```python
from build123d import *

# Parameters (mm, degrees)
BOSS_EXTRUDE1_DEPTH                                 = 10
CBORE_FOR_M5_HEX_SOCKET_HEAD_CAP_SCREW1_D           = 5.5
CBORE_FOR_M5_HEX_SOCKET_HEAD_CAP_SCREW1_CBORE_D     = 10
CBORE_FOR_M5_HEX_SOCKET_HEAD_CAP_SCREW1_CBORE_DEPTH = 8


with BuildPart() as part:
    # Sketch1 → Boss-Extrude1 (new, symmetric)
    with BuildSketch(Plane.XY):
        with BuildLine():
            Line((-15, 7.5), (-15, -7.5))
            Line((-15, -7.5), (15, -7.5))
            Line((15, -7.5), (15, 7.5))
            ThreePointArc((15, 7.5), (0, 22.5), (-15, 7.5))
        make_face()
    extrude(amount=BOSS_EXTRUDE1_DEPTH, both=True)

    # CBORE for M5 Hex Socket Head Cap Screw1 (through all)
    with Locations(Plane(origin=(0, 22.5, 0), x_dir=(1, 0, 0), z_dir=(0, 1, 0))):
        with Locations((0, 0)):
            CounterBoreHole(CBORE_FOR_M5_HEX_SOCKET_HEAD_CAP_SCREW1_D / 2, CBORE_FOR_M5_HEX_SOCKET_HEAD_CAP_SCREW1_CBORE_D / 2, CBORE_FOR_M5_HEX_SOCKET_HEAD_CAP_SCREW1_CBORE_DEPTH)


solid = part.part
```
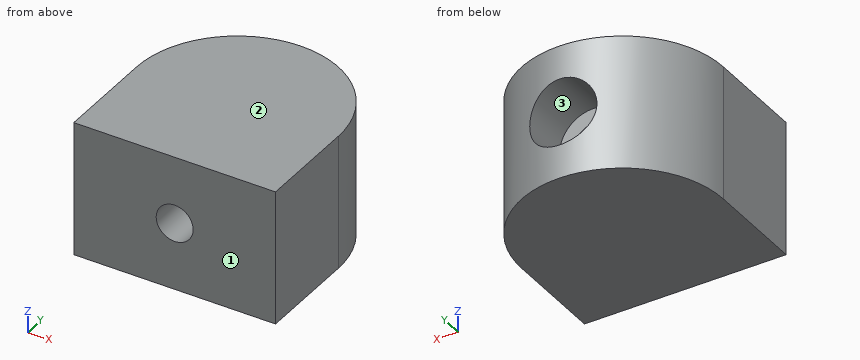
Can you work these out from the model? Positions are in its coordinate system, mm. Face numbers are marked on the shaded views. Coordinates: 2 decimals unless noted, no trailing zeros. Loops run counter-clockwise (first coordinate to the right, second up) from the corner with the lowest first, then second, coordinate; pieces in that order, holes last.
1) I need wall thicknesses on probe 1 along Z at (x, y) = (0, 8.5); probe 2 along Z at (x, y) = (0, 19); probe 3 along X at (y, z) = (16.5, -0.75). Which ranges of each line are inside material? Lowest first, please.
2) Thinking about a two-plate mould opening in Z: for the marked faces 1, 2 and 3, which applies, pulls with the +Z half, pulls with the -Z half, needs draft (parallel to the pull), parting line crosses it, or undercut?
3) For pin 1 (8 mm diameter, centred on x = -2.5, z = 0.5, fed in from +Y), with a flat end and sliding along its axis, tell me the tip position at first contact or that it passes through.
4) Imagine slicing it at B-B on y = -2. List the corners of the cut face in (x, z) for me.
5) Imagine slicing it at C-C on z = -0.5. List the corners of the cut face in (x, y) for me, plus the area to 3 significant figures.
6) Imagine slicing it at D-D on x = -3.5. List the corners of the cut face in (y, z) for me, plus the area to 3 significant figures.
7) Imagine slicing it at A-A on x = 0. List the corners of the cut face in (y, z) for me, plus the area to 3 significant figures.
Completed:
1. probe 1: z = -10 to -2.75, 2.75 to 10
1. probe 2: z = -10 to -5, 5 to 10
1. probe 3: x = -12 to -4.94, 4.94 to 12
2. face 1: needs draft
2. face 2: pulls with the +Z half
2. face 3: undercut
3. pin 1: stops at y = 22.34
4. outline: (-15, -10) - (15, -10) - (15, 10) - (-15, 10) - close; hole circle Ø5.5 at (0, 0)
5. outline: (-15, -7.5) - (-2.7, -7.5) - (-2.7, 14.5) - (-4.97, 14.5) - (-4.97, 21.65) arc R15 ccw to (-15, 7.5) - close; (2.7, -7.5) - (15, -7.5) - (15, 7.5) arc R15 ccw to (4.97, 21.65) - (4.97, 14.5) - (2.7, 14.5) - close
5. area: 608 mm2
6. outline: (-7.5, -10) - (22.09, -10) - (22.09, -3.57) - (14.5, -3.57) - (14.5, 3.57) - (22.09, 3.57) - (22.09, 10) - (-7.5, 10) - close
6. area: 538 mm2
7. outline: (-7.5, -10) - (22.5, -10) - (22.5, -5) - (14.5, -5) - (14.5, -2.75) - (-7.5, -2.75) - close; (-7.5, 2.75) - (14.5, 2.75) - (14.5, 5) - (22.5, 5) - (22.5, 10) - (-7.5, 10) - close
7. area: 399 mm2
